Here's the drawing with two shaded views (mm, measured from the low corner). I have some questions. A direction names the side the tool comes from. Give positions to 0.01 mm unless a question says otherwise; leave off trailing zeros. Write each loop counter-clockwise with the first axis right and the second up, starting at its lowest first coordinate (ties: lowest second). Pieces come first, ordered by that corner, then holes. Notation, with made-up numbers: (0.5, -13.75) -> (57.5, -13.75) arc R29 ccw to (57.5, 12.25) -> close; hole circle Ø4 at (63.5, -25.5). An arc over 180 degrees is marked (long way). One line per question, with ' | ' between items.
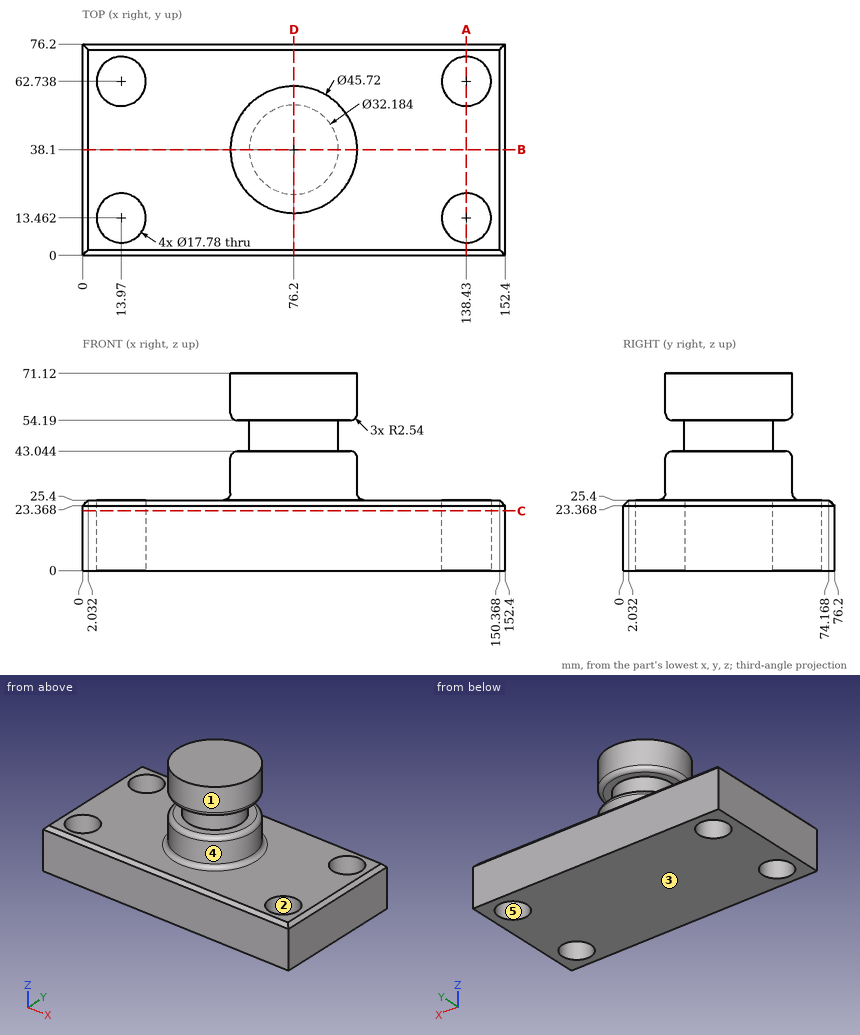
Q1. On a 3-axis mill with a long thin cutter (end or side, diameter ignored), from which of +Z, -Z, +X, -X, +Y, -Y can I reach the whole of each face in a straight line? I mean the marked faces 4 and 5. Say none if no direction works.
Answer below:
face 4: +Z | face 5: +Z, -Z
Q2. Imagine slicing it at C-C on z = 21.5. Please give me the cut outline in (x, y), and give its area (3 significant figures).
Answer below:
outline: (0, 0) -> (152.4, 0) -> (152.4, 76.2) -> (0, 76.2) -> close; hole circle Ø17.78 at (13.97, 13.46); hole circle Ø17.78 at (13.97, 62.74); hole circle Ø17.78 at (138.43, 13.46); hole circle Ø17.78 at (138.43, 62.74) | area: 10,600 mm^2
Q3. Imagine slicing it at B-B on y = 38.1. Please give me the cut outline in (x, z) (1 decimal), and give its area (3 significant figures).
Answer below:
outline: (0, 0) -> (152.4, 0) -> (152.4, 23.4) -> (150.4, 25.4) -> (101.6, 25.4) arc R2.5 cw to (99.1, 27.9) -> (99.1, 40.5) arc R2.5 ccw to (96.5, 43) -> (92.3, 43) -> (92.3, 54.2) -> (96.5, 54.2) arc R2.5 ccw to (99.1, 56.7) -> (99.1, 71.1) -> (53.3, 71.1) -> (53.3, 56.7) arc R2.5 ccw to (55.9, 54.2) -> (60.1, 54.2) -> (60.1, 43) -> (55.9, 43) arc R2.5 ccw to (53.3, 40.5) -> (53.3, 27.9) arc R2.5 cw to (50.8, 25.4) -> (2, 25.4) -> (0, 23.4) -> close | area: 5,800 mm^2
Q4. Will these pins go through, and if not, where does the flat tip stop? pin 1 (4 mm diameter, centred on x = 89, z = 45.5, fed in from +Y); pin 2 (2 mm diameter, centred on y = 14, z = 27.5, fed in from +X); pin 3 (12 mm diameter, centred on x = 91, z = 36.5, fed in from -Y); pin 4 (5 mm diameter, centred on x = 47, y = 65, fed in from +Z).
Answer below:
pin 1: stops at y = 50.03 | pin 2: passes through | pin 3: stops at y = 17 | pin 4: stops at z = 25.4
Q5. If we mould it in two halves opening along X, with no side actions, what happens to the marked faces 1, 2 and 3? For each: +X half, -X half, draft (parallel to the pull), parting line (faces both ways), or undercut.
Answer below:
face 1: parting line | face 2: undercut | face 3: draft
Q6. Imagine slicing it at D-D on x = 76.2. Please give me the cut outline in (y, z) (1 decimal).
Answer below:
outline: (0, 0) -> (76.2, 0) -> (76.2, 23.4) -> (74.2, 25.4) -> (63.5, 25.4) arc R2.5 cw to (61, 27.9) -> (61, 40.5) arc R2.5 ccw to (58.4, 43) -> (54.2, 43) -> (54.2, 54.2) -> (58.4, 54.2) arc R2.5 ccw to (61, 56.7) -> (61, 71.1) -> (15.2, 71.1) -> (15.2, 56.7) arc R2.5 ccw to (17.8, 54.2) -> (22, 54.2) -> (22, 43) -> (17.8, 43) arc R2.5 ccw to (15.2, 40.5) -> (15.2, 27.9) arc R2.5 cw to (12.7, 25.4) -> (2, 25.4) -> (0, 23.4) -> close
Q7. Imagine slicing it at A-A on x = 138.43. Please give me the cut outline in (y, z), and give its area (3 significant figures).
Answer below:
outline: (0, 0) -> (4.57, 0) -> (4.57, 25.4) -> (2.03, 25.4) -> (0, 23.37) -> close; (22.35, 0) -> (53.85, 0) -> (53.85, 25.4) -> (22.35, 25.4) -> close; (71.63, 0) -> (76.2, 0) -> (76.2, 23.37) -> (74.17, 25.4) -> (71.63, 25.4) -> close | area: 1,030 mm^2
Q8. If I drill on line 1 along Y through (x, z) = (138, 14); line 2 along Y through (x, z) = (138.43, 14.5); line 3 along Z through (x, y) = (73.5, 21) (1 decimal), over which ranges is the centre line in solid material (lowest first)?
Answer below:
line 1: y = 0 to 4.58, 22.34 to 53.86, 71.62 to 76.2 | line 2: y = 0 to 4.57, 22.35 to 53.85, 71.63 to 76.2 | line 3: z = 0 to 43, 54.2 to 71.1
